Could you check a few things on this model? Use its own coordinates, in mm. A direction names the side the tool comes from. Coordinates: 2 decimals unless noted, no trailing zeros. Write each loop counter-clockwise with the first axis right and the second up, starting at its lowest first coordinate (ties: lowest second). Pieces come first, ordered by that corner, then holes.
Item 1: Which directions (+Z, -Z, +X, -X, +Y, -Y) give clear straight access to the entire face, cutting with the end or side of a thin tool? Please do faces 4 (the cylindrical face through (21.19, 11, 23.78)), 5 (the flat face through (9, 5, 9)), 6 (the flat face through (21.25, 2, 0)).
Item 2: If I drill on probe 1 along X at (y, z) = (3.9, -15.5); probe 2 along Y at (x, z) = (-22.5, 23.9); probe 3 along Z at (x, y) = (0, 2), over which ranges is the centre line in solid material (lowest first)?
Item 3: I want a section at A-A on y = 37. Please give me the cut outline in (x, z).
Item 4: Thinking about a two-plate mould opening in Y: for faces 1 (the cylindrical face through (21.284, 38.115, 23.785)), 2 (the flat face through (0, 42, 24)), 3 (the cylindrical face through (-14.7, 2.5, -14)), which applies, +Y half, -Y half, draft (parallel to the pull), parting line (faces both ways), or undercut?
Item 5: I want a section at C-C on x = 15.5. Please give me the cut outline in (y, z).
Item 6: For P1, Ø2, axis at x = 12.5, z = 16.5, coming from the +Y side; P2, Ø1.5, axis at y = 1.5, z = -9, coming from the +X side; P3, Ø5.5, axis at y = 2, z = 2.5, coming from the -X side, each with a flat end and sliding along its axis, tell me the tip position at first contact or that it passes through.
Item 7: I want a section at B-B on z = 15.5. Please give me the cut outline in (x, y).
Item 8: I want a section at D-D on z = -10. Please give me the cut outline in (x, y).
from build123d import *

# Parameters (mm, degrees)
SKETCH1_W           = 42.5
SKETCH1_H           = 42.5
SKETCH1_R           = 1.7
SKETCH1_R_2         = 12.5
BOSS_EXTRUDE1_DEPTH = 5
SKETCH3_W           = 53
SKETCH3_H           = 5
BOSS_EXTRUDE3_DEPTH = 42
SKETCH4_R           = 1.65
CUT_EXTRUDE1_DEPTH  = 42


with BuildPart() as part:
    # Sketch1 → Boss-Extrude1 (new body)
    with BuildSketch(Plane(origin=(0, 0, 0), x_dir=(1, 0, 0), z_dir=(0, 1, 0))):
        Rectangle(SKETCH1_W, SKETCH1_H)
        with Locations((-15.5, 15.5)):
            Circle(SKETCH1_R, mode=Mode.SUBTRACT)
        with Locations((15.5, 15.5)):
            Circle(SKETCH1_R, mode=Mode.SUBTRACT)
        with Locations((-15.5, -15.5)):
            Circle(SKETCH1_R, mode=Mode.SUBTRACT)
        with Locations((15.5, -15.5)):
            Circle(SKETCH1_R, mode=Mode.SUBTRACT)
        Circle(SKETCH1_R_2, mode=Mode.SUBTRACT)
    extrude(amount=BOSS_EXTRUDE1_DEPTH)

    # Sketch3 → Boss-Extrude3 (add)
    with BuildSketch(Plane(origin=(0, 0, 0), x_dir=(1, 0, 0), z_dir=(0, 1, 0))):
        with Locations((0, -23.75)):
            Rectangle(SKETCH3_W, SKETCH3_H)
    extrude(amount=BOSS_EXTRUDE3_DEPTH)

    # Sketch4 → Cut-Extrude1 (cut)
    with BuildSketch(Plane.XY.offset(26.25)):
        with Locations((22.5, 37)):
            Circle(SKETCH4_R)
        with Locations((22.5, 12)):
            Circle(SKETCH4_R)
        with Locations((-22.5, 37)):
            Circle(SKETCH4_R)
        with Locations((-22.5, 12)):
            Circle(SKETCH4_R)
    extrude(amount=-CUT_EXTRUDE1_DEPTH, mode=Mode.SUBTRACT)


solid = part.part
Response values:
1. face 4: +Z, -Z
1. face 5: -Z, +X, -X, +Y
1. face 6: -Z, +X, +Y, -Y
2. probe 1: x = -21.25 to -17.2, -13.8 to 13.8, 17.2 to 21.25
2. probe 2: y = 0 to 10.35, 13.65 to 35.35, 38.65 to 42
2. probe 3: z = -21.25 to -12.5, 12.5 to 26.25
3. outline: (-26.5, 21.25) - (-24.15, 21.25) - (-24.15, 26.25) - (-26.5, 26.25) - close; (-20.85, 21.25) - (20.85, 21.25) - (20.85, 26.25) - (-20.85, 26.25) - close; (24.15, 21.25) - (26.5, 21.25) - (26.5, 26.25) - (24.15, 26.25) - close
4. face 1: undercut
4. face 2: +Y half
4. face 3: draft
5. outline: (0, -21.25) - (5, -21.25) - (5, -17.2) - (0, -17.2) - close; (0, -13.8) - (5, -13.8) - (5, 13.8) - (0, 13.8) - close; (0, 17.2) - (5, 17.2) - (5, 21.25) - (42, 21.25) - (42, 26.25) - (0, 26.25) - close
6. P1: stops at y = 5
6. P2: stops at x = 21.25
6. P3: stops at x = -21.25
7. outline: (-21.25, 0) - (-17.2, 0) - (-17.2, 5) - (-21.25, 5) - close; (-13.8, 0) - (13.8, 0) - (13.8, 5) - (-13.8, 5) - close; (17.2, 0) - (21.25, 0) - (21.25, 5) - (17.2, 5) - close
8. outline: (-21.25, 0) - (-7.5, 0) - (-7.5, 5) - (-21.25, 5) - close; (7.5, 0) - (21.25, 0) - (21.25, 5) - (7.5, 5) - close
